```python
from build123d import *

# Parameters (mm, degrees)
SKETCH1_W           = 20
SKETCH1_H           = 20
BOSS_EXTRUDE1_DEPTH = 100
CUT_EXTRUDE3_DEPTH  = 20
CUT_EXTRUDE4_DEPTH  = 18
FILLET3_R           = 20
SKETCH6_R           = 5
CUT_EXTRUDE5_DEPTH  = 5


with BuildPart() as part:
    # Sketch1 → Boss-Extrude1 (new body)
    with BuildSketch(Plane.XY):
        Rectangle(SKETCH1_W, SKETCH1_H)
    extrude(amount=-BOSS_EXTRUDE1_DEPTH)

    # Sketch4 → Cut-Extrude3 (cut)
    with BuildSketch(Plane(origin=(10, 0, 0), x_dir=(0, 0, -1), z_dir=(1, 0, 0))):
        Polygon((19.388888889, 10), (0, 10), (18, 5), align=None)
        Polygon((4, -10), (0, 10), (0, -10), align=None)
    extrude(amount=-CUT_EXTRUDE3_DEPTH, mode=Mode.SUBTRACT)

    # Sketch5 → Cut-Extrude4 (cut)
    with BuildSketch(Plane.XY):
        Polygon((-10, 5), (10, 10), (-10, 10), align=None)
    extrude(amount=-CUT_EXTRUDE4_DEPTH, mode=Mode.SUBTRACT)

    # Fillet3
    fillet3_edges = [part.edges().sort_by_distance(p)[0] for p in [
        (0, 7.5, -9),
    ]]
    fillet(fillet3_edges, radius=FILLET3_R)

    # Sketch6 → Cut-Extrude5 (cut)
    with BuildSketch(Plane(origin=(0, 10, 0), x_dir=(1, 0, 0), z_dir=(0, 1, 0))):
        with Locations((0, 70.114708412)):
            Circle(SKETCH6_R)
    extrude(amount=-CUT_EXTRUDE5_DEPTH, mode=Mode.SUBTRACT)


solid = part.part
```
For this review, take the finished solid that the model builds, in its own axes (mm). A direction names the side the tool comes from. Round coordinates to 2 decimals unless told otherwise and drop trailing zeros. Write each loop counter-clockwise with the first axis right and the second up, starting at its lowest first coordinate (ties: lowest second). Pieces come first, ordered by that corner, then holes.
1) Take a section at A-A on y = 6. State how many separate pieces and enclosed holes the cut face has, then the cut area to 3 significant figures.
Answer below:
separate pieces: 2
enclosed holes: 1
area: 1,770 mm2
2) Machinability: for faces 4 (the face through (2.69, 7.54, -74.33)), 5 (the face through (0.1, 7.2, -8.8)), 6 (the face through (0, 0, -2)), 7 (the face through (-4.553, 6.362, -5.189)), which of the approach directions +Z, -Z, +X, -X, +Y, -Y give a long, thin tool a straight path to every point of the face, cutting with its end or side? Answer none if there is none.
Answer below:
face 4: +Y
face 5: -X, +Y
face 6: +Z, +X, -X, -Y
face 7: +Z, -X, +Y
3) Take a section at B-B on y = -6. Give the boundary of the cut face in (x, z), then the cut area to 3 significant figures.
Answer below:
outline: (-10, -100) - (10, -100) - (10, -3.2) - (-10, -3.2) - close
area: 1,940 mm2
4) Insertion check: pin 1 Ø2 at (x, y) = (0, -7) entering from +Z; pin 2 Ø5 at (x, z) = (-1, -71.5) entering from +Y; pin 3 Ø1.5 at (x, y) = (-6, 2) entering from +Z. Each pin has a flat end and moves straight along its axis. Give the tip position at first contact, or say it passes through.
Answer below:
pin 1: stops at z = -3.2
pin 2: stops at y = 5
pin 3: stops at z = -1.45
5) Mouldability with a two-part tool opening along Z and no side actions: class faces 1 (the face through (0, 0, -100)), 2 (the face through (10, 0, -49)), 3 (the face through (6.04, 6.04, -14.25)) as +Z half, -Z half, draft (parallel to the pull), parting line (faces both ways), or undercut.
Answer below:
face 1: -Z half
face 2: draft
face 3: undercut
6) For line 1 along Z through (x, y) = (0, 7.85); line 2 along Z through (x, y) = (0, 8.9); line 3 along Y through (x, z) = (-4.5, -71), list the stretches that pass through material, from the lowest coordinate up.
Answer below:
line 1: z = -100 to -75.11, -65.11 to -18.79
line 2: z = -100 to -75.11, -65.11 to -19.08
line 3: y = -10 to 5
